Input: part model. Units: mm. Frame: model coordinates. Face numbers are marked on the shaded views. Give positions to 0.01 mm unless a question says otherwise; leave off trailing zeros. Loops run counter-clockwise (first coordinate to the right, second up) from the corner with the lowest first, then second, coordinate; pieces in that order, holes last. Notation, with made-up numbers: M -33,-22.75 L 24,-22.75 A22 cw 24,14.25 Z; hole C 5,55.25 d8. An arc over 180 degrees is marked long. Use CSV: the item, a comma, the result in double quotes. Start each with the question number.
Q1. Section D-D, the plane y = -5. Output: boundary loops of the cut face in (x, z), plus the area to 3 significant figures.
Q2. Section C-C, the plane z = 32. Output: boundary loops of the cut face in (x, y).
Q3. Material intervals for line 1 along X through (y, z) = (-50, 1.7); line 2 along Y through (x, z) = (20, 3.15); line 3 along X through (y, z) = (-6, 33.5), sorted ascending.
Q4. Section A-A, the plane x = 10. Output: boundary loops of the cut face in (y, z).
Q5. Section B-B, the plane z = 24. Output: boundary loops of the cut face in (x, y).
Q6. Pin query (flat end, axial travel): pin 1 (1.5 mm diameter, centred on x = 19, z = 47.5, fed in from -Y); pin 2 (8 mm diameter, centred on x = -0.5, y = -48, fed in from +Z); pin 3 (2 mm diameter, centred on x = -1, y = -11.5, fed in from +Z). Return the tip coordinate at first contact, or that it passes through.
Q7. Pull-direction query (X, two-part tool) for the marked faces 1, 2 and 3; classes: released by +X, released by -X, zero draft, split by the parting line, or undercut.
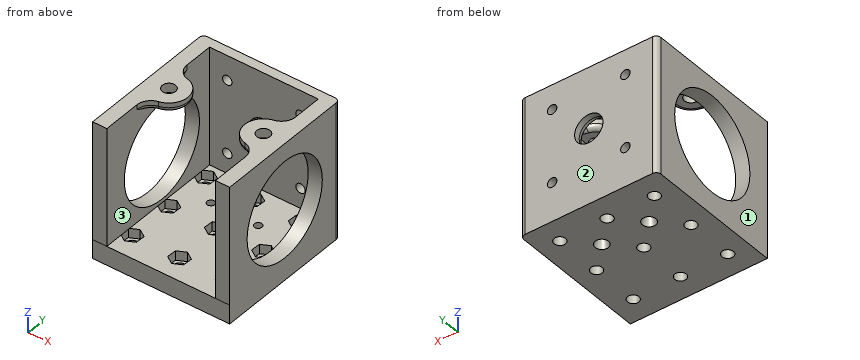
from build123d import *
from OCP.BRepFilletAPI import BRepFilletAPI_MakeChamfer

# Parameters (mm, degrees)
SKIZZE1_W                       = 58
SKIZZE1_H                       = 60
SKIZZE1_R                       = 2.4
SKIZZE1_R_2                     = 1.6
AUFSATZ_LINEAR_AUSTRAGEN1_DEPTH = 8
AUFSATZ_LINEAR_AUSTRAGEN2_DEPTH = 50
SKIZZE5_R                       = 6
SKIZZE5_R_2                     = 2
SCHNITT_LINEAR_AUSTRAGEN1_DEPTH = 8
SKIZZE10_R                      = 8
SKIZZE10_R_2                    = 2.8
AUFSATZ_LINEAR_AUSTRAGEN3_DEPTH = 4
VERRUNDUNG1_R                   = 6
VERRUNDUNG3_R                   = 2
SKIZZE11_R                      = 2.8
SCHNITT_LINEAR_AUSTRAGEN7_DEPTH = 4
FASE3_SIZE                      = 0.4
FASE3_SIZE2                     = 1.492820323
VERRUNDUNG4_R                   = 2
FASE4_SIZE                      = 4.5
FASE4_SIZE2                     = 1.205771366
SCHNITT_LINEAR_AUSTRAGEN8_DEPTH = 4
LINEARES_MUSTER1_COUNT          = 3
LINEARES_MUSTER1_PITCH          = 20
LINEARES_MUSTER1_COUNT_DIR2     = 3
LINEARES_MUSTER1_PITCH_DIR2     = 20
SKIZZE13_R                      = 20.5
SCHNITT_LINEAR_AUSTRAGEN9_DEPTH = 60


with BuildPart() as part:
    # Skizze1 → Aufsatz-Linear austragen1 (new body)
    with BuildSketch(Plane.XY):
        with Locations((0, -30)):
            Rectangle(SKIZZE1_W, SKIZZE1_H)
        with Locations((-20, -10)):
            Circle(SKIZZE1_R, mode=Mode.SUBTRACT)
        with Locations((0, -10)):
            Circle(SKIZZE1_R, mode=Mode.SUBTRACT)
        with Locations((20, -10)):
            Circle(SKIZZE1_R, mode=Mode.SUBTRACT)
        with Locations((0, -30)):
            Circle(SKIZZE1_R, mode=Mode.SUBTRACT)
        with Locations((20, -30)):
            Circle(SKIZZE1_R, mode=Mode.SUBTRACT)
        with Locations((0, -50)):
            Circle(SKIZZE1_R, mode=Mode.SUBTRACT)
        with Locations((20, -50)):
            Circle(SKIZZE1_R, mode=Mode.SUBTRACT)
        with Locations((-20, -30)):
            Circle(SKIZZE1_R, mode=Mode.SUBTRACT)
        with Locations((-20, -50)):
            Circle(SKIZZE1_R, mode=Mode.SUBTRACT)
        with Locations((-10, -20)):
            Circle(SKIZZE1_R_2, mode=Mode.SUBTRACT)
        with Locations((10, -20)):
            Circle(SKIZZE1_R_2, mode=Mode.SUBTRACT)
    extrude(amount=AUFSATZ_LINEAR_AUSTRAGEN1_DEPTH)

    # Skizze4 → Aufsatz-Linear austragen2 (add)
    with BuildSketch(Plane.XY.offset(8)):
        Polygon((29, 0), (-29, 0), (-29, -59.997453527), (-23, -59.997453527), (-23, -4), (23, -4), (23, -59.997453527), (29, -59.997453527), align=None)
    extrude(amount=AUFSATZ_LINEAR_AUSTRAGEN2_DEPTH)

    # Skizze5 → Schnitt-Linear austragen1 (cut)
    with BuildSketch(Plane(origin=(0, 0, 0), x_dir=(1, 0, 0), z_dir=(0, 1, 0))):
        with Locations(Location((0, -32, 0), (0, 0, 180))):
            Circle(SKIZZE5_R)
        with Locations(Location((-15.5, -16.5, 0), (0, 0, 180))):
            Circle(SKIZZE5_R_2)
        with Locations(Location((15.5, -16.5, 0), (0, 0, 180))):
            Circle(SKIZZE5_R_2)
        with Locations(Location((15.5, -47.5, 0), (0, 0, 180))):
            Circle(SKIZZE5_R_2)
        with Locations(Location((-15.5, -47.5, 0), (0, 0, 180))):
            Circle(SKIZZE5_R_2)
    extrude(amount=-SCHNITT_LINEAR_AUSTRAGEN1_DEPTH, mode=Mode.SUBTRACT)

    # Skizze10 → Aufsatz-Linear austragen3 (add)
    # profile 1 of 2: a face of its own
    with BuildSketch(Plane.XY.offset(58)):
        with Locations((20, -30)):
            Circle(SKIZZE10_R)
    # profile 2 of 2: a face of its own
    with BuildSketch(Plane.XY.offset(58)):
        with Locations((-20, -30)):
            Circle(SKIZZE10_R)
        with Locations((-20, -30)):
            Circle(SKIZZE10_R_2, mode=Mode.SUBTRACT)
    extrude(amount=-AUFSATZ_LINEAR_AUSTRAGEN3_DEPTH)

    # Verrundung1
    verrundung1_edges = [part.edges().sort_by_distance(p)[0] for p in [
        (23, -37.416198487, 56),
        (23, -22.583801513, 56),
        (-23, -37.416198487, 56),
        (-23, -22.583801513, 56),
    ]]
    fillet(verrundung1_edges, radius=VERRUNDUNG1_R)

    # Verrundung3
    # the kernel refuses this fillet: 2 mm, written as the material it takes off along each edge
    with BuildSketch(Plane(origin=(-20, -30, 54), x_dir=(0.21428571428571433, -0.9767710236555245, 0), z_dir=(-0.9767710236555245, -0.21428571428571433, 0))) as verrundung3_piece_1:
        with BuildLine():
            CenterArc((8 - VERRUNDUNG3_R, VERRUNDUNG3_R), VERRUNDUNG3_R, 270, 90)
            Line((8 - VERRUNDUNG3_R, 0), (8, 0))
            Line((8, 0), (8, VERRUNDUNG3_R))
        make_face()
    revolve(axis=Axis((-20, -30, 54), (0, 0, 1)), revolution_arc=155.252749768, mode=Mode.SUBTRACT)
    with BuildSketch(Plane(origin=(20, -30, 54), x_dir=(-0.21428571428571347, 0.9767710236555247, 0), z_dir=(0.9767710236555247, 0.21428571428571347, 0))) as verrundung3_piece_2:
        with BuildLine():
            CenterArc((8 - VERRUNDUNG3_R, VERRUNDUNG3_R), VERRUNDUNG3_R, 270, 90)
            Line((8 - VERRUNDUNG3_R, 0), (8, 0))
            Line((8, 0), (8, VERRUNDUNG3_R))
        make_face()
    revolve(axis=Axis((20, -30, 54), (0, 0, 1)), revolution_arc=155.252749768, mode=Mode.SUBTRACT)
    with BuildSketch(Plane(origin=(-17, -16.325205669, 54), x_dir=(-0.6722279054593165, 0.7403442733767718, 0), z_dir=(0.7403442733767718, 0.6722279054593165, 0))) as verrundung3_piece_3_section:
        with BuildLine():
            CenterArc((6 + VERRUNDUNG3_R, VERRUNDUNG3_R), VERRUNDUNG3_R, 180, 90)
            Line((6 + VERRUNDUNG3_R, 0), (6, 0))
            Line((6, 0), (6, VERRUNDUNG3_R))
        make_face()
    verrundung3_piece_3 = revolve(axis=Axis((-17, -16.325205669, 54), (0, 0, 1)), revolution_arc=125.387125524, mode=Mode.PRIVATE)
    verrundung3_piece_3 = split(verrundung3_piece_3, bisect_by=Plane(origin=(-23, -20.355034942, 54.516064296), z_dir=(1, 0, 0)), keep=Keep.TOP, mode=Mode.PRIVATE)
    add(verrundung3_piece_3, mode=Mode.SUBTRACT)
    with BuildSketch(Plane(origin=(-17, -43.674794331, 54), x_dir=(-0.6722279054593165, -0.7403442733767718, 0), z_dir=(0.7403442733767718, -0.6722279054593165, 0))) as verrundung3_piece_4_section:
        with BuildLine():
            CenterArc((6 + VERRUNDUNG3_R, -VERRUNDUNG3_R), VERRUNDUNG3_R, 90, 90)
            Line((6, -VERRUNDUNG3_R), (6, 0))
            Line((6, 0), (6 + VERRUNDUNG3_R, 0))
        make_face()
    verrundung3_piece_4 = revolve(axis=Axis((-17, -43.674794331, 54), (0, 0, -1)), revolution_arc=125.387125524, mode=Mode.PRIVATE)
    verrundung3_piece_4 = split(verrundung3_piece_4, bisect_by=Plane(origin=(-23, -39.644965239, 54.51606418), z_dir=(1, 0, 0)), keep=Keep.TOP, mode=Mode.PRIVATE)
    add(verrundung3_piece_4, mode=Mode.SUBTRACT)
    with BuildSketch(Plane(origin=(17, -43.674794331, 54), x_dir=(0.6722279054593165, -0.7403442733767718, 0), z_dir=(-0.7403442733767718, -0.6722279054593165, 0))) as verrundung3_piece_5_section:
        with BuildLine():
            CenterArc((6 + VERRUNDUNG3_R, VERRUNDUNG3_R), VERRUNDUNG3_R, 180, 90)
            Line((6 + VERRUNDUNG3_R, 0), (6, 0))
            Line((6, 0), (6, VERRUNDUNG3_R))
        make_face()
    verrundung3_piece_5 = revolve(axis=Axis((17, -43.674794331, 54), (0, 0, 1)), revolution_arc=125.387125524, mode=Mode.PRIVATE)
    verrundung3_piece_5 = split(verrundung3_piece_5, bisect_by=Plane(origin=(23, -39.644965059, 54.516064297), z_dir=(-1, 0, 0)), keep=Keep.TOP, mode=Mode.PRIVATE)
    add(verrundung3_piece_5, mode=Mode.SUBTRACT)
    with BuildSketch(Plane(origin=(17, -16.325205669, 54), x_dir=(0.6722279054593165, 0.7403442733767718, 0), z_dir=(-0.7403442733767718, 0.6722279054593165, 0))) as verrundung3_piece_6_section:
        with BuildLine():
            CenterArc((6 + VERRUNDUNG3_R, -VERRUNDUNG3_R), VERRUNDUNG3_R, 90, 90)
            Line((6, -VERRUNDUNG3_R), (6, 0))
            Line((6, 0), (6 + VERRUNDUNG3_R, 0))
        make_face()
    verrundung3_piece_6 = revolve(axis=Axis((17, -16.325205669, 54), (0, 0, -1)), revolution_arc=125.387125524, mode=Mode.PRIVATE)
    verrundung3_piece_6 = split(verrundung3_piece_6, bisect_by=Plane(origin=(23, -20.355037545, 54.516064214), z_dir=(-1, 0, 0)), keep=Keep.TOP, mode=Mode.PRIVATE)
    add(verrundung3_piece_6, mode=Mode.SUBTRACT)

    # Skizze11 → Schnitt-Linear austragen7 (cut)
    with BuildSketch(Plane.XY.offset(58)):
        with Locations((20, -30)):
            Circle(SKIZZE11_R)
    extrude(amount=-SCHNITT_LINEAR_AUSTRAGEN7_DEPTH, mode=Mode.SUBTRACT)

    # Fase3
    fase3_edges = [part.edges().sort_by_distance(p)[0] for p in [
        (6, -4, 32),
    ]]
    fase3_side = [part.faces().sort_by_distance(p)[0] for p in [
        (-22.32058849, -4, 33),
    ]]
    chamfer(fase3_edges, length=FASE3_SIZE, length2=FASE3_SIZE2, reference=fase3_side[0])

    # Verrundung4
    verrundung4_edges = [part.edges().sort_by_distance(p)[0] for p in [
        (-29, 0, 29),
        (29, 0, 29),
    ]]
    fillet(verrundung4_edges, radius=VERRUNDUNG4_R)

    # Fase4: one chamfer whose edges measure the first distance from different faces: ONE call of the kernel's chamfer builder (chamfer() names one face for all edges)
    fase4_edges_1 = [part.edges().sort_by_distance(p)[0] for p in [
        (-11.6, -20, 0),
    ]]
    fase4_side_1 = [part.faces().sort_by_distance(p)[0] for p in [
        (-11.6, -20, 4),
    ]]
    fase4_edges_2 = [part.edges().sort_by_distance(p)[0] for p in [
        (8.4, -20, 0),
    ]]
    fase4_side_2 = [part.faces().sort_by_distance(p)[0] for p in [
        (8.4, -20, 4),
    ]]
    fase4 = BRepFilletAPI_MakeChamfer(part.part.solid().wrapped)
    for e in fase4_edges_1:
        fase4.Add(FASE4_SIZE, FASE4_SIZE2, e.wrapped, fase4_side_1[0].wrapped)  # the first distance lies on this face
    for e in fase4_edges_2:
        fase4.Add(FASE4_SIZE, FASE4_SIZE2, e.wrapped, fase4_side_2[0].wrapped)  # the first distance lies on this face
    add(Compound.cast(fase4.Shape()), mode=Mode.REPLACE)

    # Skizze12 → Schnitt-Linear austragen8 (cut)
    with BuildSketch(Plane.XY.offset(8)):
        Polygon((-16.6027319, -12.189041523), (-16.405600381, -8.152400284), (-19.802868481, -5.96335876), (-23.3972681, -7.810958477), (-23.594399619, -11.847599716), (-20.197131519, -14.03664124), align=None)
    schnitt_linear_austragen8 = extrude(amount=-SCHNITT_LINEAR_AUSTRAGEN8_DEPTH, mode=Mode.SUBTRACT)

    # Lineares Muster1: Schnitt-Linear austragen8 3 × 3
    with Locations(*[(i * LINEARES_MUSTER1_PITCH, -j * LINEARES_MUSTER1_PITCH_DIR2, 0) for i in range(LINEARES_MUSTER1_COUNT) for j in range(LINEARES_MUSTER1_COUNT_DIR2) if (i, j) != (0, 0)]):
        add(schnitt_linear_austragen8, mode=Mode.SUBTRACT)

    # Skizze13 → Schnitt-Linear austragen9 (cut)
    with BuildSketch(Plane(origin=(29, 0, 0), x_dir=(0, 0, -1), z_dir=(1, 0, 0))):
        with Locations(Location((-30, -30, 0), (0, 0, 90))):
            Circle(SKIZZE13_R)
    extrude(amount=-SCHNITT_LINEAR_AUSTRAGEN9_DEPTH, mode=Mode.SUBTRACT)


solid = part.part
A:
1,outline,"M -29,0 L 29,0 L 29,58 L 23,58 L 23,8 L -23,8 L -23,58 L -29,58 Z"
1,area,"1,060 mm^2"
2,outline,"M -29,-60 L -23,-60 L -23,-50.4 L -29,-50.4 Z; M -29,-9.6 L -23,-9.6 L -23,-4 L -6.4,-4 L -6,-2.51 L -6,0 L -27,0 A2 ccw -29,-2 Z; M 6,-2.51 L 6.4,-4 L 23,-4 L 23,-9.6 L 29,-9.6 L 29,-2 A2 ccw 27,0 L 6,0 Z; M 23,-60 L 29,-60 L 29,-50.4 L 23,-50.4 Z"
3,line 1,"-29 to -22.4, -17.6 to -2.4, 2.4 to 17.6, 22.4 to 29"
3,line 2,"-60 to -52.4, -47.6 to -32.4, -27.6 to -12.4, -7.6 to 0"
3,line 3,"-29 to -23, 23 to 29"
4,outline,"M -60,0 L -22.81,0 L -21.6,4.5 L -21.6,8 L -60,8 Z; M -18.4,4.5 L -17.19,0 L 0,0 L 0,58 L -4,58 L -4,8 L -18.4,8 Z"
5,outline,"M -29,-60 L -23,-60 L -23,-49.6 L -29,-49.6 Z; M -29,-10.4 L -23,-10.4 L -23,-4 L 23,-4 L 23,-10.4 L 29,-10.4 L 29,-2 A2 ccw 27,0 L -27,0 A2 ccw -29,-2 Z; M 23,-60 L 29,-60 L 29,-49.6 L 23,-49.6 Z"
6,pin 1,"y = -4"
6,pin 2,"z = 8"
6,pin 3,"z = 4"
7,face 1,"released by -X"
7,face 2,"zero draft"
7,face 3,"undercut"
